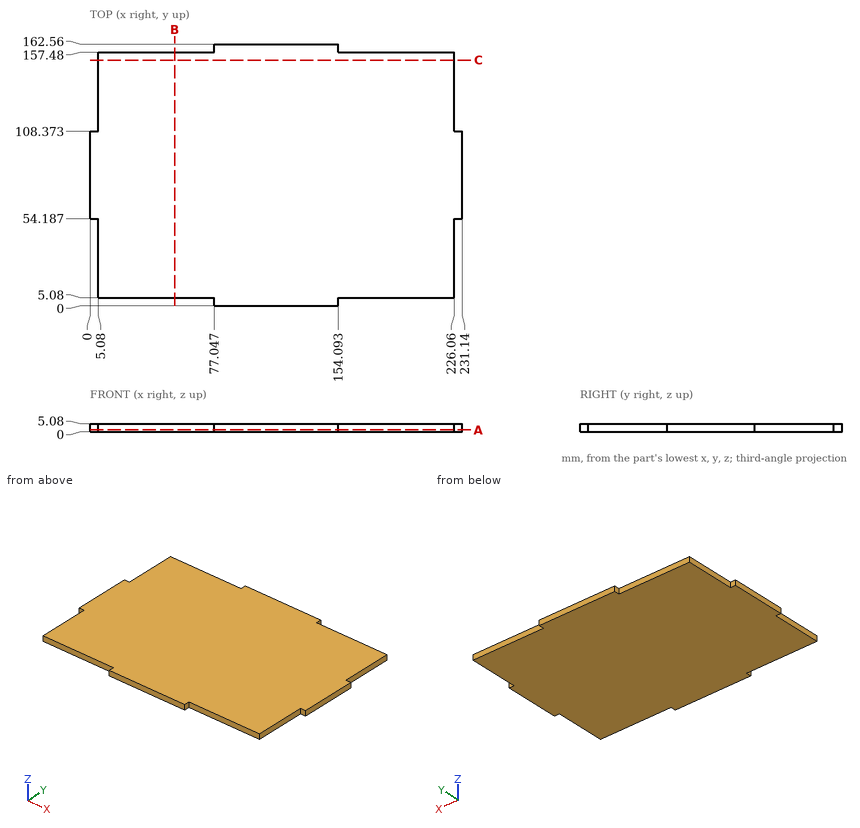
The figure shows three views and two pictorial views of one solid part (mm, origin at its lowest corner). Answer the questions. Coordinates: 2 decimals unless noted, no trailing zeros. Order: outer loops, then holes, each group sorted by start corner. A loop starts at its lowest first (then second) coordinate and runs counter-clockwise, first axis right, second up.
Q1. Consider line 1 (X direction, y = 134.5, z = 2.75); line 2 (Y direction, x = 163, z = 1.15). Determine where each line is inside the solid, lowest interval first.
Q2. A cutting plane is placed at C-C, the plane y = 152.5. Write down the section's boundary in (x, z), and give its area (3 significant figures).
Q3. A cutting plane is placed at B-B, the plane x = 52.5. Write down the section's boundary in (y, z).
Q4. Given P1, Ø2.5, axis at x = 3, z = 2, coming from the +Y side; P2, Ø2.5, axis at y = 21.5, z = 1.5, coming from the +X side; P3, Ø1.5, axis at y = 3.5, z = 3.5, coming from the +X side, each flat-ended and moving along its own axis, determine where each tip first touches the part or whether it passes through.
Q5. A cutting plane is placed at A-A, the plane z = 1.3. Write down the section's boundary in (x, y).
Answers follow:
1. line 1: x = 5.08 to 226.06
1. line 2: y = 5.08 to 157.48
2. outline: (5.08, 0) - (226.06, 0) - (226.06, 5.08) - (5.08, 5.08) - close
2. area: 1,120 mm2
3. outline: (5.08, 0) - (157.48, 0) - (157.48, 5.08) - (5.08, 5.08) - close
4. P1: stops at y = 108.37
4. P2: stops at x = 226.06
4. P3: stops at x = 154.09
5. outline: (0, 54.19) - (5.08, 54.19) - (5.08, 5.08) - (77.05, 5.08) - (77.05, 0) - (154.09, 0) - (154.09, 5.08) - (226.06, 5.08) - (226.06, 54.19) - (231.14, 54.19) - (231.14, 108.37) - (226.06, 108.37) - (226.06, 157.48) - (154.09, 157.48) - (154.09, 162.56) - (77.05, 162.56) - (77.05, 157.48) - (5.08, 157.48) - (5.08, 108.37) - (0, 108.37) - close
